from build123d import *

# Parameters (mm, degrees)
SKETCH1_R           = 1.5
SKETCH1_R_2         = 3
BOSS_EXTRUDE1_DEPTH = 2.5
SKETCH2_W           = 15
SKETCH2_H           = 2.5
CUT_EXTRUDE1_DEPTH  = 3
CUT_EXTRUDE2_DEPTH  = 3
SKETCH4_W           = 2.5
SKETCH4_H           = 9
CUT_EXTRUDE3_DEPTH  = 12
SKETCH5_W           = 15
SKETCH5_H           = 10
CUT_EXTRUDE4_DEPTH  = 2.5


with BuildPart() as part:
    # Sketch1 → Boss-Extrude1 (new body)
    with BuildSketch(Plane.XY):
        Polygon((87, 23), (106.918584287, 11.5), (106.918584287, -11.5), (87, -23), (-87, -23), (-106.918584287, -11.5), (-106.918584287, 11.5), (-87, 23), align=None)
        with Locations((43.5, -14.8)):
            Circle(SKETCH1_R, mode=Mode.SUBTRACT)
        with Locations((-43.5, 2.8)):
            Circle(SKETCH1_R, mode=Mode.SUBTRACT)
        with Locations((-43.5, -14.8)):
            Circle(SKETCH1_R, mode=Mode.SUBTRACT)
        with Locations((-64, -6)):
            Circle(SKETCH1_R_2, mode=Mode.SUBTRACT)
        with Locations((43.5, 2.8)):
            Circle(SKETCH1_R, mode=Mode.SUBTRACT)
        with Locations((64, -6)):
            Circle(SKETCH1_R_2, mode=Mode.SUBTRACT)
    extrude(amount=BOSS_EXTRUDE1_DEPTH)

    # Sketch2 → Cut-Extrude1 (cut)
    with BuildSketch(Plane.XY.offset(2.5)):
        with Locations((-63.5, 19.75)):
            Rectangle(SKETCH2_W, SKETCH2_H)
        with Locations((-63.5, -19.75)):
            Rectangle(SKETCH2_W, SKETCH2_H)
        with Locations((63.5, -19.75)):
            Rectangle(SKETCH2_W, SKETCH2_H)
        with Locations((63.5, 19.75)):
            Rectangle(SKETCH2_W, SKETCH2_H)
    extrude(amount=-CUT_EXTRUDE1_DEPTH, mode=Mode.SUBTRACT)

    # Sketch3 → Cut-Extrude2 (cut)
    with BuildSketch(Plane.XY.offset(2.5)):
        Polygon((-90.151279442, 18.871206889), (-88.901279442, 16.70614338), (-99.293584287, 10.70614338), (-100.543584287, 12.871206889), align=None)
        Polygon((-88.901279442, -16.70614338), (-90.151279442, -18.871206889), (-100.543584287, -12.871206889), (-99.293584287, -10.70614338), align=None)
        Polygon((99.293584287, -10.70614338), (100.543584287, -12.871206889), (90.151279442, -18.871206889), (88.901279442, -16.70614338), align=None)
        Polygon((100.543584287, 12.871206889), (99.293584287, 10.70614338), (88.901279442, 16.70614338), (90.151279442, 18.871206889), align=None)
    extrude(amount=-CUT_EXTRUDE2_DEPTH, mode=Mode.SUBTRACT)

    # Sketch4 → Cut-Extrude3 (cut)
    with BuildSketch(Plane.XY.offset(2.5)):
        with Locations((-103.668584287, 0)):
            Rectangle(SKETCH4_W, SKETCH4_H)
        with Locations((103.668584287, 0)):
            Rectangle(SKETCH4_W, SKETCH4_H)
    extrude(amount=-CUT_EXTRUDE3_DEPTH, mode=Mode.SUBTRACT)

    # Sketch5 → Cut-Extrude4 (cut)
    with BuildSketch(Plane.XY.offset(2.5)):
        with Locations((0, 13)):
            Rectangle(SKETCH5_W, SKETCH5_H)
    extrude(amount=-CUT_EXTRUDE4_DEPTH, mode=Mode.SUBTRACT)


solid = part.part
Geometry: final body of the model. Coordinates: model frame, mm. A direction names the side the tool comes from. Give positions to 0.01 mm unless a question says otherwise; leave off trailing zeros. Loops run counter-clockwise (first coordinate to the right, second up) from the corner with the lowest first, then second, coordinate; pieces in that order, holes last. Notation, with made-up numbers: M -34.75,89.5 L 24.25,89.5 A13 ccw 24.25,111.5 Z; hole C -13.5,67.5 d4. An arc over 180 degrees is marked long. Put each result on its own line as item: value. Start each with the question number.
1) Cut plane C-C (z = 1.9). Give the number of separate pieces and of enclosed holes in the cut face, then the cut area to 3 significant figures.
2) Cut plane A-A (x = 64). Output: boundary loops of the cut face in (y, z).
3) Cut plane B-B (x = 0). Output: boundary loops of the cut face in (y, z).
4) Contact query for flat-ended pins moving along their axis: pin 1 (1 mm diameter, centred on y = -13.5, z = 2, fed in from -X); pin 2 (0.8 mm diameter, centred on x = -104, z = 1, fed in from +Y); pin 3 (3.5 mm diameter, centred on x = 64, y = -6, fed in from +Z). Output: stop coordinate, or through.
5) Pull-direction query (Y, two-part tool) for faces 1 (the flat face through (96.82, 17.33, 1.23)), 2 (the flat face through (95.42, -15.83, 1.27)), 3 (the flat face through (-96.82, -17.33, 1.23)); classes: pulls with the +Y half, pulls with the -Y half, needs draft (parallel to the pull), parting line crosses it, or undercut.
6) Access query for faces 4 (the flat face through (95.3, 15.9, 1.3)), 5 (the flat face through (1, 0, 2.5)). Directions: +Z, -Z, +X, -X, +Y, -Y. A direction counts if a zero-diameter tool reaches every point of the face in a straight line with its end or side. Return the directions, or none.
7) Ray query, line 1 along Y through (x, z) = (-43.5, 0.7); line 2 along X through (y, z) = (-1.5, 0.65); line 3 along X through (y, z) = (-6.5, 0.4). Return the intervals inside material, ascending.
Verdict:
1. separate pieces: 1
1. enclosed holes: 17
1. area: 8,830 mm2
2. outline: M -23,0 L -21,0 L -21,2.5 L -23,2.5 Z; M -18.5,0 L -9,0 L -9,2.5 L -18.5,2.5 Z; M -3,0 L 18.5,0 L 18.5,2.5 L -3,2.5 Z; M 21,0 L 23,0 L 23,2.5 L 21,2.5 Z
3. outline: M -23,0 L 8,0 L 8,2.5 L -23,2.5 Z; M 18,0 L 23,0 L 23,2.5 L 18,2.5 Z
4. pin 1: x = -104.32
4. pin 2: y = 13.42
4. pin 3: through
5. face 1: pulls with the +Y half
5. face 2: undercut
5. face 3: pulls with the -Y half
6. face 4: +Z, -Z
6. face 5: +Z, +X, -X, +Y, -Y
7. line 1: -23 to -16.3, -13.3 to 1.3, 4.3 to 23
7. line 2: -106.92 to -104.92, -102.42 to 102.42, 104.92 to 106.92
7. line 3: -106.92 to -66.96, -61.04 to 61.04, 66.96 to 106.92
